```python
from build123d import *

# Parameters (mm, degrees)
F0_W     = 50.8
F0_H     = 101.6
F0_R     = 7.62
F1_DEPTH = 12.7
F2_R     = 5.08
F3_R     = 2.39168
F4_DEPTH = 72.39


with BuildPart() as f1:
    # F0 (on Front) → F1 (new body, symmetric)
    with BuildSketch(Plane.XZ):
        Rectangle(F0_W, F0_H)
        with Locations((0, -26.461581)):
            Circle(F0_R, mode=Mode.SUBTRACT)
        with Locations((0, 26.461581)):
            Circle(F0_R, mode=Mode.SUBTRACT)
    extrude(amount=F1_DEPTH, both=True)

    # F2
    f2_edges = [f1.edges().sort_by_distance(p)[0] for p in [
        (-25.4, 0, 50.8),
        (25.4, 0, 50.8),
        (25.4, 0, -50.8),
        (-25.4, 0, -50.8),
    ]]
    fillet(f2_edges, radius=F2_R)

    # F3 (on face) → F4 (cut, symmetric)
    with BuildSketch(Plane.XZ.offset(12.7)):
        with Locations((-20.32, 45.72)):
            Circle(F3_R)
        with Locations((20.32, 45.72)):
            Circle(F3_R)
        with Locations((20.32, -45.72)):
            Circle(F3_R)
        with Locations((-20.32, -45.72)):
            Circle(F3_R)
    extrude(amount=F4_DEPTH, both=True, mode=Mode.SUBTRACT)


solid = f1.part
```
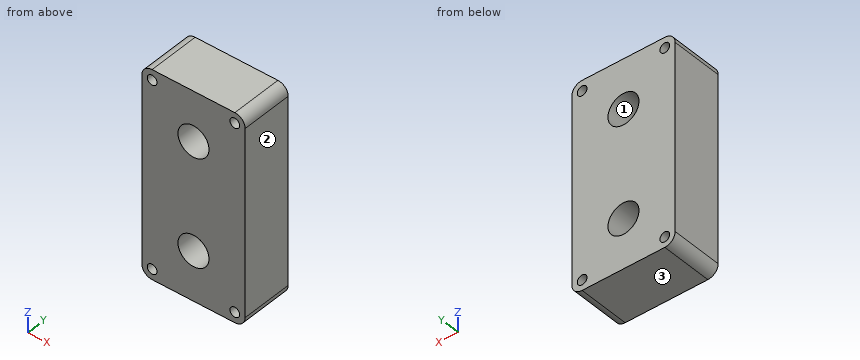
Input: part model. Units: mm. Frame: model coordinates. Face numbers are marked on the shaded views. Coordinates: 2 decimals unless noted, no trailing zeros. Write each loop counter-clockwise with the first axis right and the second up, starting at its lowest first coordinate (ties: lowest second). Pieces come first, ordered by that corner, then holes.
1) Section A-A on x = -6. Output: boundary loops of the cut face in (y, z).
2) Section D-D on x = 5.5. Output: boundary loops of the cut face in (y, z), and give its area (3 significant figures).
3) Material intervals for line 1 along Z through (x, y) = (0, -1); line 2 along Z through (x, y) = (0.5, 3.75); line 3 along X through (y, z) = (-9.75, -20.5), sorted ascending.
4) Section C-C on y = 8.25. Output: boundary loops of the cut face in (x, z).
5) Mould query, pull axis X, two halves, no side actions, for the marked faces 1, 2 and 3. Classes: pulls with the +X half, pulls with the -X half, needs draft (parallel to the pull), parting line crosses it, or undercut.
6) Pin query (flat end, axial travel): pin 1 Ø17.5 at (x, z) = (0, 26.46) entering from +Y. Return the tip coordinate at first contact, or that it passes through.
7) Section B-B on z = -21.5. Output: boundary loops of the cut face in (x, y), and give its area (3 significant figures).
Check result:
1. outline: (-12.7, -50.8) - (12.7, -50.8) - (12.7, -31.16) - (-12.7, -31.16) - close; (-12.7, -21.76) - (12.7, -21.76) - (12.7, 21.76) - (-12.7, 21.76) - close; (-12.7, 31.16) - (12.7, 31.16) - (12.7, 50.8) - (-12.7, 50.8) - close
2. outline: (-12.7, -50.8) - (12.7, -50.8) - (12.7, -31.74) - (-12.7, -31.74) - close; (-12.7, -21.19) - (12.7, -21.19) - (12.7, 21.19) - (-12.7, 21.19) - close; (-12.7, 31.74) - (12.7, 31.74) - (12.7, 50.8) - (-12.7, 50.8) - close
2. area: 2,040 mm2
3. line 1: z = -50.8 to -34.08, -18.84 to 18.84, 34.08 to 50.8
3. line 2: z = -50.8 to -34.07, -18.86 to 18.86, 34.07 to 50.8
3. line 3: x = -25.4 to -4.75, 4.75 to 25.4
4. outline: (-25.4, -45.72) arc R5.08 ccw to (-20.32, -50.8) - (20.32, -50.8) arc R5.08 ccw to (25.4, -45.72) - (25.4, 45.72) arc R5.08 ccw to (20.32, 50.8) - (-20.32, 50.8) arc R5.08 ccw to (-25.4, 45.72) - close; hole circle Ø4.78 at (-20.32, -45.72); hole circle Ø4.78 at (-20.32, 45.72); hole circle Ø15.24 at (0, -26.46); hole circle Ø15.24 at (0, 26.46); hole circle Ø4.78 at (20.32, -45.72); hole circle Ø4.78 at (20.32, 45.72)
5. face 1: undercut
5. face 2: pulls with the +X half
5. face 3: needs draft
6. pin 1: stops at y = 12.7
7. outline: (-25.4, -12.7) - (-5.78, -12.7) - (-5.78, 12.7) - (-25.4, 12.7) - close; (5.78, -12.7) - (25.4, -12.7) - (25.4, 12.7) - (5.78, 12.7) - close
7. area: 997 mm2
